CAD build for the part. Positions are in the model's coordinates, mm. Face numbers are marked on the shaded views. Round coordinates to 2 decimals unless told otherwise and drop trailing zeros. Order: outer loops, then holes, each group sorted by start corner. A loop starts at its lowest first (then second) coordinate and runs counter-clockwise, first axis right, second up.
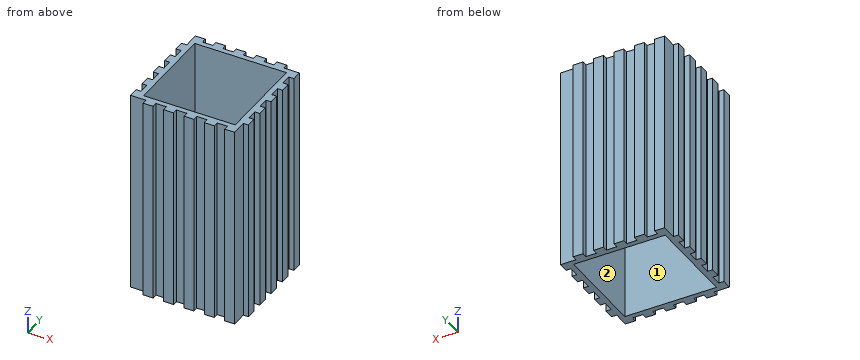
```python
from build123d import *

# Parameters (mm, degrees)
SKETCH_W  = 90
SKETCH_H  = 90
PAD_DEPTH = 200


with BuildPart() as part:
    # Sketch → Pad (new body)
    with BuildSketch(Plane.XY):
        Polygon((-50, 55), (-40.25, 55), (-40.25, 50), (-30, 50), (-30, 55), (-20.25, 55), (-20.25, 50), (-10, 50), (-10, 55), (-0.25, 55), (-0.25, 50), (10, 50), (10, 55), (19.75, 55), (19.75, 50), (30, 50), (30, 55), (39.75, 55), (39.75, 50), (50, 50), (55, 50), (55, 40.25), (50, 40.25), (50, 30), (55, 30), (55, 20.25), (50, 20.25), (50, 10), (55, 10), (55, 0.25), (50, 0.25), (50, -10), (55, -10), (55, -19.75), (50, -19.75), (50, -30), (55, -30), (55, -39.75), (50, -39.75), (50, -50), (50, -55), (40.25, -55), (40.25, -50), (30, -50), (30, -55), (20.25, -55), (20.25, -50), (10, -50), (10, -55), (0.25, -55), (0.25, -50), (-10, -50), (-10, -55), (-19.75, -55), (-19.75, -50), (-30, -50), (-30, -55), (-39.75, -55), (-39.75, -50), (-50, -50), (-55, -50), (-55, -40.25), (-50, -40.25), (-50, -30), (-55, -30), (-55, -20.25), (-50, -20.25), (-50, -10), (-55, -10), (-55, -0.25), (-50, -0.25), (-50, 10), (-55, 10), (-55, 19.75), (-50, 19.75), (-50, 30), (-55, 30), (-55, 39.75), (-50, 39.75), (-50, 50), align=None)
        Rectangle(SKETCH_W, SKETCH_H, mode=Mode.SUBTRACT)
    extrude(amount=PAD_DEPTH)


solid = part.part
```
1. Drill centre lines: line 1 (Y direction, x = 34.5, z = 43); line 2 (X direction, y = 17, z = 39). Where is each one in solid material? Low to high.
2. Mould opens along Y. For the marked faces 1 and 2 say: released by +Y, released by -Y, zero draft, split by the parting line, or undercut.
3. Cut at A-A, the plane x = -25.5. Write the cut outline in (y, z), and give its area (3 significant figures).
4. Pin check, flat tips, straight feed: P1, Ø3, axis at x = 13.5, z = 56.5, coming from the -Y side; P2, Ø7.5, axis at x = 47, z = 101, coming from the +Y side; P3, Ø5.5, axis at y = 53, z = 144.5, coming from the -X side; P4, Ø10, axis at x = -39, y = -6.5, coming from the -Z side. Stop position of each tip, or through.
Outcome:
1. line 1: y = -50 to -45, 45 to 55
1. line 2: x = -55 to -45, 45 to 50
2. face 1: undercut
2. face 2: undercut
3. outline: (-50, 0) - (-45, 0) - (-45, 200) - (-50, 200) - close; (45, 0) - (55, 0) - (55, 200) - (45, 200) - close
3. area: 3,000 mm2
4. P1: stops at y = -50
4. P2: stops at y = 50
4. P3: stops at x = -50
4. P4: passes through
